Can you work these out from the model? Positions are in its coordinate system, mm. A direction names the side the tool comes from. Coordinates: 2 decimals unless noted, no trailing zeros. Loops run counter-clockwise (first coordinate to the right, second up) from the corner with the lowest first, then second, coordinate; pieces in that order, holes last. Notation, with made-up numbers: (20.5, 20.5) -> (50.5, 20.5) arc R29 ccw to (50.5, 51.5) -> close; hole circle Ø1 at (35, 75.25). An arc over 180 degrees is marked (long way). Put each result on its own line as item: value. Start each with the question number.
Item 1: If we section it at B-B on x = -19.05: Please give me the cut outline in (y, z).
Item 2: If we section it at D-D on z = -52.07: Please give me the cut outline in (x, y).
Item 3: For faces 4 (the flat face through (-133.096, 2, -70)), 5 (the flat face through (-3.175, 2, -38)), 6 (the flat face through (-120, 2, -62.307)), which set-ups out of +Z, -Z, +X, -X, +Y, -Y let a thin tool reach every point of the face, with its end or its side?
Item 4: Will this pin go through, and if not, where does the flat tip stop? P1, Ø1.7, axis at y = 1, z = -33, coming from the +X side (3 decimals).
Item 5: If we section it at C-C on z = -19.05: Please give me the cut outline in (x, y), plus the area to 3 significant figures.
Item 6: We'd pull the mould along Z, two halves only. Please class faces 1 (the flat face through (-2, 2, -27.305)), 2 (the flat face through (-81, 0, -30)), 3 (the flat face through (-83, 2, -76.2)): pulls with the +Z half, pulls with the -Z half, needs draft (parallel to the pull), parting line crosses it, or undercut.
Item 7: If we section it at A-A on z = -66.04: Please give me the cut outline in (x, y), plus the area to 3 significant figures.
Item 8: Please list where these lines run through material, in increasing order: L1, parallel to X at y = 1, z = -52; L2, parallel to X at y = 1.8, z = -9.5; L3, parallel to X at y = 2.35, z = -57.15. Write a range as from..to.
```python
from build123d import *

# Parameters (mm, degrees)
SKETCH1_R           = 1.8288
BOSS_EXTRUDE1_DEPTH = 3.302
SKETCH2_R           = 1.524
CUT_EXTRUDE1_DEPTH  = 4.302
SKETCH3_R           = 1.375
CUT_EXTRUDE2_DEPTH  = 4.302
SKETCH4_W           = 3.175
SKETCH4_H           = 10.16
SKETCH4_W_2         = 10.16
SKETCH4_H_2         = 3.175
CUT_EXTRUDE3_DEPTH  = 4.302
SKETCH5_R           = 1.524
CUT_EXTRUDE4_DEPTH  = 4.302


with BuildPart() as part:
    # Sketch1 → Boss-Extrude1 (new body)
    with BuildSketch(Plane(origin=(0, 0, 0), x_dir=(1, 0, 0), z_dir=(0, 1, 0))):
        Polygon((-164.846, 76.2), (-139.446, 76.2), (-139.446, 63.5), (-133.096, 63.5), (-133.096, 76.2), (-31.75, 76.2), (-31.75, 63.5), (-25.4, 63.5), (-25.4, 76.2), (0, 76.2), (0, 48.895), (-3.175, 48.895), (-3.175, 27.305), (0, 27.305), (0, 0), (-25.4, 0), (-25.4, 12.7), (-31.75, 12.7), (-31.75, 0), (-133.096, 0), (-133.096, 12.7), (-139.446, 12.7), (-139.446, 0), (-164.846, 0), (-164.846, 27.305), (-164.846, 48.895), align=None)
        with Locations((-82.423, 38.1)):
            Circle(SKETCH1_R, mode=Mode.SUBTRACT)
    extrude(amount=BOSS_EXTRUDE1_DEPTH)

    # Sketch2 → Cut-Extrude1 (cut, through all)
    with BuildSketch(Plane(origin=(0, 3.302, 0), x_dir=(1, 0, 0), z_dir=(0, 1, 0))):
        with Locations((-159.766, 66.04)):
            Circle(SKETCH2_R)
        with Locations((-128.016, 66.04)):
            Circle(SKETCH2_R)
        with Locations((-128.016, 52.07)):
            Circle(SKETCH2_R)
        with Locations((-159.766, 52.07)):
            Circle(SKETCH2_R)
    extrude(amount=-CUT_EXTRUDE1_DEPTH, mode=Mode.SUBTRACT)

    # Sketch3 → Cut-Extrude2 (cut, through all)
    with BuildSketch(Plane(origin=(0, 3.302, 0), x_dir=(1, 0, 0), z_dir=(0, 1, 0))):
        with Locations((-154.686, 6.35)):
            Circle(SKETCH3_R)
        with Locations((-115.186, 6.35)):
            Circle(SKETCH3_R)
        with Locations((-115.186, 25.85)):
            Circle(SKETCH3_R)
        with Locations((-154.686, 25.85)):
            Circle(SKETCH3_R)
    extrude(amount=-CUT_EXTRUDE2_DEPTH, mode=Mode.SUBTRACT)

    # Sketch4 → Cut-Extrude3 (cut, through all)
    with BuildSketch(Plane(origin=(0, 3.302, 0), x_dir=(1, 0, 0), z_dir=(0, 1, 0))):
        with Locations((-65.63129104, 67.386847386)):
            Rectangle(SKETCH4_W, SKETCH4_H)
        with Locations((-95.06194853, 43.1165)):
            Rectangle(SKETCH4_W_2, SKETCH4_H_2)
        with Locations((-119.60629104, 67.386847386)):
            Rectangle(SKETCH4_W, SKETCH4_H)
    extrude(amount=-CUT_EXTRUDE3_DEPTH, mode=Mode.SUBTRACT)

    # Sketch5 → Cut-Extrude4 (cut, through all)
    with BuildSketch(Plane(origin=(0, 3.302, 0), x_dir=(1, 0, 0), z_dir=(0, 1, 0))):
        with Locations((-19.05, 19.05)):
            Circle(SKETCH5_R)
        with Locations((-19.05, 57.15)):
            Circle(SKETCH5_R)
    extrude(amount=-CUT_EXTRUDE4_DEPTH, mode=Mode.SUBTRACT)


solid = part.part
```
Solutions:
1. outline: (0, -76.2) -> (3.3, -76.2) -> (3.3, -58.67) -> (0, -58.67) -> close; (0, -55.63) -> (3.3, -55.63) -> (3.3, -20.57) -> (0, -20.57) -> close; (0, -17.53) -> (3.3, -17.53) -> (3.3, 0) -> (0, 0) -> close
2. outline: (-164.85, 0) -> (-161.29, 0) -> (-161.29, 3.3) -> (-164.85, 3.3) -> close; (-158.24, 0) -> (-129.54, 0) -> (-129.54, 3.3) -> (-158.24, 3.3) -> close; (-126.49, 0) -> (0, 0) -> (0, 3.3) -> (-126.49, 3.3) -> close
3. face 4: -Z, +Y, -Y
3. face 5: +X, +Y, -Y
3. face 6: +Y, -Y
4. P1: x = -3.175
5. outline: (-164.85, 0) -> (-20.57, 0) -> (-20.57, 3.3) -> (-164.85, 3.3) -> close; (-17.53, 0) -> (0, 0) -> (0, 3.3) -> (-17.53, 3.3) -> close
5. area: 534 mm^2
6. face 1: undercut
6. face 2: needs draft
6. face 3: pulls with the -Z half
7. outline: (-164.85, 0) -> (-161.29, 0) -> (-161.29, 3.3) -> (-164.85, 3.3) -> close; (-158.24, 0) -> (-139.45, 0) -> (-139.45, 3.3) -> (-158.24, 3.3) -> close; (-133.1, 0) -> (-129.54, 0) -> (-129.54, 3.3) -> (-133.1, 3.3) -> close; (-126.49, 0) -> (-121.19, 0) -> (-121.19, 3.3) -> (-126.49, 3.3) -> close; (-118.02, 0) -> (-67.22, 0) -> (-67.22, 3.3) -> (-118.02, 3.3) -> close; (-64.04, 0) -> (-31.75, 0) -> (-31.75, 3.3) -> (-64.04, 3.3) -> close; (-25.4, 0) -> (0, 0) -> (0, 3.3) -> (-25.4, 3.3) -> close
7. area: 461 mm^2
8. L1: -164.85..-161.29, -158.24..-129.54, -126.49..0
8. L2: -164.85..-139.45, -133.1..-31.75, -25.4..0
8. L3: -164.85..-20.57, -17.53..0
